from build123d import *

# Parameters (mm, degrees)
BOSS_EXTRUDE1_DEPTH  = 7
SKETCH6_W            = 5
SKETCH6_H            = 10
BOSS_EXTRUDE2_DEPTH  = 4
SKETCH3_W            = 5.1
SKETCH3_H            = 7.5
CUT_EXTRUDE1_DEPTH   = 4
M4_CLEARANCE_HOLE1_D = 4.5
CHAMFER2_SIZE        = 4
CHAMFER5_SIZE        = 0.5


# Some blends are built 0.0001 mm under size
with BuildPart() as part:
    # Sketch1 → Boss-Extrude1 (new body)
    with BuildSketch(Plane.XY):
        Polygon((0, 0), (0, -10), (-19, -10), (-21.5, -12.5), (-21.5, -27.5), (-26.5, -27.5), (-26.5, -7.5), (-19, 0), align=None)
    boss_extrude1 = extrude(amount=BOSS_EXTRUDE1_DEPTH)

    # Sketch6 → Boss-Extrude2 (add)
    with BuildSketch(Plane.XY.offset(7)):
        with Locations((-24, -22.5)):
            Rectangle(SKETCH6_W, SKETCH6_H)
    boss_extrude2 = extrude(amount=BOSS_EXTRUDE2_DEPTH)

    # Sketch3 → Cut-Extrude1 (cut)
    with BuildSketch(Plane.XY.offset(7)):
        with Locations((-2.55, -3.75)):
            Rectangle(SKETCH3_W, SKETCH3_H)
    cut_extrude1 = extrude(amount=-CUT_EXTRUDE1_DEPTH, mode=Mode.SUBTRACT)

    # Mirror1: Boss-Extrude1, Boss-Extrude2, Cut-Extrude1 across plane
    add(boss_extrude1.mirror(Plane(origin=(0, 0, 7), x_dir=(0, 0, 1), z_dir=(-1, 0, 0))))
    add(boss_extrude2.mirror(Plane(origin=(0, 0, 7), x_dir=(0, 0, 1), z_dir=(-1, 0, 0))))
    add(cut_extrude1.mirror(Plane(origin=(0, 0, 7), x_dir=(0, 0, 1), z_dir=(-1, 0, 0))), mode=Mode.SUBTRACT)

    # M4 Clearance Hole1 (through all)
    with Locations(Plane.XY.offset(3)):
        with Locations((0, -3.5)):
            Hole(M4_CLEARANCE_HOLE1_D / 2)

    # Chamfer2
    chamfer2_edges = [part.edges().sort_by_distance(p)[0] for p in [
        (-24, -17.5, 7),
        (24, -17.5, 7),
    ]]
    chamfer(chamfer2_edges, length=CHAMFER2_SIZE - 0.0001)  # a hair under: the kernel refuses the full size

    # Chamfer4
    # the kernel refuses this chamfer: 1 mm, written as the material it takes off along each edge
    with BuildSketch(Plane(origin=(26.5, -11.68164552, 5.18154552), x_dir=(-0.9996219169112968, 0.019442520806014118, 0.01944252080601436), z_dir=(0, -0.7071067811865476, 0.7071067811865476))) as chamfer4_piece_1_section:
        with BuildLine():
            Line((1.028673195, 0), (-0.056547155, 1.027117794))
            Line((-0.056547155, 1.027117794), (-0.076539593, 1.026567876))
            ThreePointArc((-0.076539593, 1.026567876), (-0.034129227, 0.51339783), (-0.019992438, -0.000549918))
            Line((-0.019992438, -0.000549918), (0.000549918, -0.019992438))
            ThreePointArc((0.000549918, -0.019992438), (0.514497665, -0.00585565), (1.029223113, -0.019992438))
            Line((1.029223113, -0.019992438), (1.028673195, 0))
        make_face()
    chamfer4_piece_1 = extrude(amount=10.800078804, mode=Mode.PRIVATE)
    chamfer4_piece_1 = split(chamfer4_piece_1, bisect_by=Plane(origin=(26.156619069, -15.715277747, 7), z_dir=(0, 0, 1)), keep=Keep.TOP, mode=Mode.PRIVATE)
    add(chamfer4_piece_1, mode=Mode.SUBTRACT)
    with BuildSketch(Plane(origin=(-26.5, -11.68164552, 5.18154552), x_dir=(0.9996219169112968, 0.019442520806013806, 0.019442520806013806), z_dir=(0, -0.7071067811865476, 0.7071067811865476))) as chamfer4_piece_2_section:
        with BuildLine():
            Line((1.028673195, 0), (-0.056547155, -1.027117794))
            Line((-0.056547155, -1.027117794), (-0.076539593, -1.026567876))
            ThreePointArc((-0.076539593, -1.026567876), (-0.034129227, -0.51339783), (-0.019992438, 0.000549918))
            Line((-0.019992438, 0.000549918), (0.000549918, 0.019992438))
            ThreePointArc((0.000549918, 0.019992438), (0.514497665, 0.00585565), (1.029223113, 0.019992438))
            Line((1.029223113, 0.019992438), (1.028673195, 0))
        make_face()
    chamfer4_piece_2 = extrude(amount=10.800078804, mode=Mode.PRIVATE)
    chamfer4_piece_2 = split(chamfer4_piece_2, bisect_by=Plane(origin=(-26.156619069, -15.715277747, 7), z_dir=(0, 0, 1)), keep=Keep.TOP, mode=Mode.PRIVATE)
    add(chamfer4_piece_2, mode=Mode.SUBTRACT)
    with BuildSketch(Plane(origin=(-28.31845448, -9.31845448, 7), x_dir=(0.7068394360706726, -0.7068394360706746, 0.027495876610586528), z_dir=(0.7071067811865485, 0.7071067811865466, 0))) as chamfer4_piece_3:
        with BuildLine():
            Line((1.028673195, 0), (-0.056547155, 1.027117794))
            Line((-0.056547155, 1.027117794), (-0.076539593, 1.026567876))
            ThreePointArc((-0.076539593, 1.026567876), (-0.034129227, 0.51339783), (-0.019992438, -0.000549918))
            Line((-0.019992438, -0.000549918), (0.000549918, -0.019992438))
            ThreePointArc((0.000549918, -0.019992438), (0.514497665, -0.00585565), (1.029223113, -0.019992438))
            Line((1.029223113, -0.019992438), (1.028673195, 0))
        make_face()
    extrude(amount=15.749967694, mode=Mode.SUBTRACT)
    with BuildSketch(Plane(origin=(-26.5, -16.071782988, 7), x_dir=(0.9996219169112968, 0, 0.02749587661058651), z_dir=(0, 1, 0))) as chamfer4_piece_4_section:
        with BuildLine():
            Line((1.028673195, 0), (-0.056547155, 1.027117794))
            Line((-0.056547155, 1.027117794), (-0.076539593, 1.026567876))
            ThreePointArc((-0.076539593, 1.026567876), (-0.034129227, 0.51339783), (-0.019992438, -0.000549918))
            Line((-0.019992438, -0.000549918), (0.000549918, -0.019992438))
            ThreePointArc((0.000549918, -0.019992438), (0.514497665, -0.00585565), (1.029223113, -0.019992438))
            Line((1.029223113, -0.019992438), (1.028673195, 0))
        make_face()
    chamfer4_piece_4 = extrude(amount=11.143465976, mode=Mode.PRIVATE)
    chamfer4_piece_4 = split(chamfer4_piece_4, bisect_by=Plane(origin=(-26.166087376, -11.115587602, 4.615487602), z_dir=(0, 0.7071067811865476, 0.7071067811865476)), keep=Keep.TOP, mode=Mode.PRIVATE)
    add(chamfer4_piece_4, mode=Mode.SUBTRACT)
    with BuildSketch(Plane(origin=(-21.571682988, 0, 7), x_dir=(0, -0.9996219169112968, 0.027495876610586494), z_dir=(1, 0, 0))) as chamfer4_piece_5:
        with BuildLine():
            Line((1.028673195, 0), (-0.056547155, 1.027117794))
            Line((-0.056547155, 1.027117794), (-0.076539593, 1.026567876))
            ThreePointArc((-0.076539593, 1.026567876), (-0.034129227, 0.51339783), (-0.019992438, -0.000549918))
            Line((-0.019992438, -0.000549918), (0.000549918, -0.019992438))
            ThreePointArc((0.000549918, -0.019992438), (0.514497665, -0.00585565), (1.029223113, -0.019992438))
            Line((1.029223113, -0.019992438), (1.028673195, 0))
        make_face()
    extrude(amount=19.043365976, mode=Mode.SUBTRACT)
    with BuildSketch(Plane(origin=(26.5, -16.071782988, 7), x_dir=(-0.9996219169112968, 0, 0.02749587661058651), z_dir=(0, 1, 0))) as chamfer4_piece_6_section:
        with BuildLine():
            Line((1.028673195, 0), (-0.056547155, -1.027117794))
            Line((-0.056547155, -1.027117794), (-0.076539593, -1.026567876))
            ThreePointArc((-0.076539593, -1.026567876), (-0.034129227, -0.51339783), (-0.019992438, 0.000549918))
            Line((-0.019992438, 0.000549918), (0.000549918, 0.019992438))
            ThreePointArc((0.000549918, 0.019992438), (0.514497665, 0.00585565), (1.029223113, 0.019992438))
            Line((1.029223113, 0.019992438), (1.028673195, 0))
        make_face()
    chamfer4_piece_6 = extrude(amount=11.143465976, mode=Mode.PRIVATE)
    chamfer4_piece_6 = split(chamfer4_piece_6, bisect_by=Plane(origin=(26.166087376, -11.115587602, 4.615487602), z_dir=(0, 0.7071067811865476, 0.7071067811865476)), keep=Keep.TOP, mode=Mode.PRIVATE)
    add(chamfer4_piece_6, mode=Mode.SUBTRACT)
    with BuildSketch(Plane(origin=(28.31845448, -9.31845448, 7), x_dir=(-0.7068394360706725, -0.7068394360706747, 0.027495876610586528), z_dir=(-0.7071067811865487, 0.7071067811865464, 0))) as chamfer4_piece_7:
        with BuildLine():
            Line((1.028673195, 0), (-0.056547155, -1.027117794))
            Line((-0.056547155, -1.027117794), (-0.076539593, -1.026567876))
            ThreePointArc((-0.076539593, -1.026567876), (-0.034129227, -0.51339783), (-0.019992438, 0.000549918))
            Line((-0.019992438, 0.000549918), (0.000549918, 0.019992438))
            ThreePointArc((0.000549918, 0.019992438), (0.514497665, 0.00585565), (1.029223113, 0.019992438))
            Line((1.029223113, 0.019992438), (1.028673195, 0))
        make_face()
    extrude(amount=15.749967694, mode=Mode.SUBTRACT)
    with BuildSketch(Plane(origin=(21.571682988, 0, 7), x_dir=(0, -0.9996219169112968, 0.027495876610586494), z_dir=(-1, 0, 0))) as chamfer4_piece_8:
        with BuildLine():
            Line((1.028673195, 0), (-0.056547155, -1.027117794))
            Line((-0.056547155, -1.027117794), (-0.076539593, -1.026567876))
            ThreePointArc((-0.076539593, -1.026567876), (-0.034129227, -0.51339783), (-0.019992438, 0.000549918))
            Line((-0.019992438, 0.000549918), (0.000549918, 0.019992438))
            ThreePointArc((0.000549918, 0.019992438), (0.514497665, 0.00585565), (1.029223113, 0.019992438))
            Line((1.029223113, 0.019992438), (1.028673195, 0))
        make_face()
    extrude(amount=19.043365976, mode=Mode.SUBTRACT)
    with BuildSketch(Plane(origin=(26.5, -16.071782988, 7), x_dir=(-0.9996219169112968, 0, 0.02749587661058651), z_dir=(0, 1, 0))) as chamfer4_piece_9a_section:
        with BuildLine():
            Line((1.028673195, 0), (-0.056547155, -1.027117794))
            Line((-0.056547155, -1.027117794), (-0.076539593, -1.026567876))
            ThreePointArc((-0.076539593, -1.026567876), (-0.034129227, -0.51339783), (-0.019992438, 0.000549918))
            Line((-0.019992438, 0.000549918), (0.000549918, 0.019992438))
            ThreePointArc((0.000549918, 0.019992438), (0.514497665, 0.00585565), (1.029223113, 0.019992438))
            Line((1.029223113, 0.019992438), (1.028673195, 0))
        make_face()
    chamfer4_piece_9a = extrude(amount=11.143465976, mode=Mode.PRIVATE)
    chamfer4_piece_9a = split(chamfer4_piece_9a, bisect_by=Plane(origin=(26.181906875, -13.879260813, 7.379160813), z_dir=(0, -0.7071067811865476, -0.7071067811865476)), keep=Keep.TOP, mode=Mode.PRIVATE)
    with BuildSketch(Plane(origin=(26.5, -11.68164552, 5.18154552), x_dir=(-0.9996219169112968, 0.019442520806014118, 0.01944252080601436), z_dir=(0, -0.7071067811865476, 0.7071067811865476))) as chamfer4_piece_9b_section:
        with BuildLine():
            Line((1.028673195, 0), (-0.056547155, 1.027117794))
            Line((-0.056547155, 1.027117794), (-0.076539593, 1.026567876))
            ThreePointArc((-0.076539593, 1.026567876), (-0.034129227, 0.51339783), (-0.019992438, -0.000549918))
            Line((-0.019992438, -0.000549918), (0.000549918, -0.019992438))
            ThreePointArc((0.000549918, -0.019992438), (0.514497665, -0.00585565), (1.029223113, -0.019992438))
            Line((1.029223113, -0.019992438), (1.028673195, 0))
        make_face()
    chamfer4_piece_9b = extrude(amount=10.800078804, mode=Mode.PRIVATE)
    chamfer4_piece_9b = split(chamfer4_piece_9b, bisect_by=Plane(origin=(26.181906875, -12.963885635, 7), z_dir=(0, 0, -1)), keep=Keep.TOP, mode=Mode.PRIVATE)
    chamfer4_piece_9 = chamfer4_piece_9a & chamfer4_piece_9b
    add(chamfer4_piece_9, mode=Mode.SUBTRACT)
    with BuildSketch(Plane(origin=(-26.5, -16.071782988, 7), x_dir=(0.9996219169112968, 0, 0.02749587661058651), z_dir=(0, 1, 0))) as chamfer4_piece_10a_section:
        with BuildLine():
            Line((1.028673195, 0), (-0.056547155, 1.027117794))
            Line((-0.056547155, 1.027117794), (-0.076539593, 1.026567876))
            ThreePointArc((-0.076539593, 1.026567876), (-0.034129227, 0.51339783), (-0.019992438, -0.000549918))
            Line((-0.019992438, -0.000549918), (0.000549918, -0.019992438))
            ThreePointArc((0.000549918, -0.019992438), (0.514497665, -0.00585565), (1.029223113, -0.019992438))
            Line((1.029223113, -0.019992438), (1.028673195, 0))
        make_face()
    chamfer4_piece_10a = extrude(amount=11.143465976, mode=Mode.PRIVATE)
    chamfer4_piece_10a = split(chamfer4_piece_10a, bisect_by=Plane(origin=(-26.181906875, -13.879260813, 7.379160813), z_dir=(0, -0.7071067811865476, -0.7071067811865476)), keep=Keep.TOP, mode=Mode.PRIVATE)
    with BuildSketch(Plane(origin=(-26.5, -11.68164552, 5.18154552), x_dir=(0.9996219169112968, 0.019442520806013806, 0.019442520806013806), z_dir=(0, -0.7071067811865476, 0.7071067811865476))) as chamfer4_piece_10b_section:
        with BuildLine():
            Line((1.028673195, 0), (-0.056547155, -1.027117794))
            Line((-0.056547155, -1.027117794), (-0.076539593, -1.026567876))
            ThreePointArc((-0.076539593, -1.026567876), (-0.034129227, -0.51339783), (-0.019992438, 0.000549918))
            Line((-0.019992438, 0.000549918), (0.000549918, 0.019992438))
            ThreePointArc((0.000549918, 0.019992438), (0.514497665, 0.00585565), (1.029223113, 0.019992438))
            Line((1.029223113, 0.019992438), (1.028673195, 0))
        make_face()
    chamfer4_piece_10b = extrude(amount=10.800078804, mode=Mode.PRIVATE)
    chamfer4_piece_10b = split(chamfer4_piece_10b, bisect_by=Plane(origin=(-26.181906875, -12.963885635, 7), z_dir=(0, 0, -1)), keep=Keep.TOP, mode=Mode.PRIVATE)
    chamfer4_piece_10 = chamfer4_piece_10a & chamfer4_piece_10b
    add(chamfer4_piece_10, mode=Mode.SUBTRACT)

    # Chamfer5
    chamfer5_edges = [part.edges().sort_by_distance(p)[0] for p in [
        (-24, -27.5, 11),
        (24, -27.5, 11),
    ]]
    chamfer(chamfer5_edges, length=CHAMFER5_SIZE)


solid = part.part
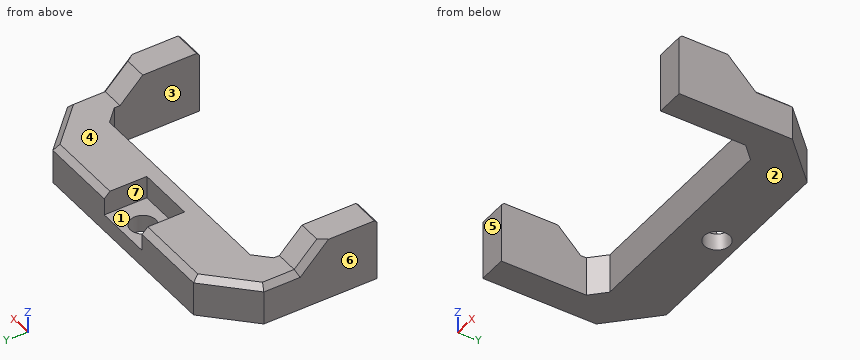
Can you work these out from the model? Positions are in its coordinate system, mm. Face numbers are marked on the shaded views. A direction names the side the tool comes from. Give positions to 0.01 mm unless a question says otherwise; leave off trailing zeros. Loops run counter-clockwise (first coordinate to the right, second up) from the corner with the lowest first, then second, coordinate; pieces in that order, holes last. Notation, with made-up numbers: (-23.5, 18) - (12.5, 18) arc R21 ccw to (12.5, 56) - close; hole circle Ø1 at (3.25, -38). An arc over 180 degrees is marked (long way). Return JSON: item names as keys, results as strings.
1. We'd pull the mould along X, two halves only. Please class the marked faces 5, 6 and 7: +X half, -X half, draft (parallel to the pull), parting line (faces both ways), or undercut.
Output values:
{"face 5": "draft", "face 6": "-X half", "face 7": "undercut"}
2. I want a section at A-A on y = -19.5. Please give me the cut outline in (x, z).
Output values:
{"outline": "(-26.5, 0) - (-21.5, 0) - (-21.5, 11) - (-26.5, 11) - close; (21.5, 0) - (26.5, 0) - (26.5, 11) - (21.5, 11) - close"}
3. For the marked faces 1, 2, 3 and 4, which set-ups out of +Z, -Z, +X, -X, +Y, -Y let a thin tool reach every point of the face, with its end or its side?
Output values:
{"face 1": "+Z, +Y", "face 2": "-Z, +X, -X, +Y, -Y", "face 3": "+Z, -Z, -Y", "face 4": "+Z, +X, -X, +Y"}
4. I want a section at D-D on x = 6.5. Please give me the cut outline in (y, z), and give its area (3 significant figures).
Output values:
{"outline": "(-10, 0) - (0, 0) - (0, 6) - (-1, 7) - (-10, 7) - close", "area": "69.5 mm²"}
5. If I drill on line 1 (Y direction, x = 0, z = 2.2); line 2 (X direction, y = -13, z = 3.5); line 3 (Z direction, x = 1, y = -1.25), over which ranges is the centre line in solid material (lowest first)?
Output values:
{"line 1": "y = -10 to -5.75, -1.25 to 0", "line 2": "x = -26.5 to -21.5, 21.5 to 26.5", "line 3": "z = 0 to 3"}
6. I want a section at C-C on z = 5.5. Please give me the cut outline in (x, y).
Output values:
{"outline": "(-26.5, -27.5) - (-21.5, -27.5) - (-21.5, -12.5) - (-19, -10) - (19, -10) - (21.5, -12.5) - (21.5, -27.5) - (26.5, -27.5) - (26.5, -7.5) - (19, 0) - (5.1, 0) - (5.1, -7.5) - (-5.1, -7.5) - (-5.1, 0) - (-19, 0) - (-26.5, -7.5) - close"}
7. I want a section at B-B on x = 0. Please give me the cut outline in (y, z).
Output values:
{"outline": "(-10, 0) - (-5.75, 0) - (-5.75, 3) - (-7.5, 3) - (-7.5, 7) - (-10, 7) - close; (-1.25, 0) - (0, 0) - (0, 3) - (-1.25, 3) - close"}
8. I'm going to push flat-ended pins straight in: pin 1 Ø5 at (y, z) = (-6.5, 9) entering from +X; pin 2 Ø2 at (x, z) = (2, 5.5) entering from +Y; pin 3 Ø6 at (x, z) = (-5.5, 3) entering from -Y. Where does each tip first touch, or does it pass through?
Output values:
{"pin 1": "stops at x = 25.59", "pin 2": "stops at y = -7.5", "pin 3": "stops at y = -10"}
